```python
from build123d import *

# Parameters (mm, degrees)
SKETCH_1_R          = 3.2
SKETCH_1_R_2        = 1.8
SKETCH_1_R_3        = 5.7
SKETCH_1_R_4        = 1.7
EXTRUDE_1_DEPTH     = 3
SKETCH_2_R          = 10.5
EXTRUDE_2_DEPTH     = 7
SKETCH_4_R          = 1.7
CUT_EXTRUDE_1_DEPTH = 7
CUT_EXTRUDE_2_DEPTH = 3.5
SKETCH_6_R          = 5.7
CUT_EXTRUDE_3_DEPTH = 20
SKETCH_7_R          = 5
SKETCH_7_R_2        = 3.2
EXTRUDE_3_DEPTH     = 15
SKETCH_8_W          = 10
SKETCH_8_H          = 4
SKETCH_8_W_2        = 4
SKETCH_8_H_2        = 6
EXTRUDE_4_DEPTH     = 15
CUT_EXTRUDE_4_DEPTH = 15
CUT_EXTRUDE_5_DEPTH = 15
CUT_EXTRUDE_6_DEPTH = 15
SKETCH_12_W         = 25.575378798
SKETCH_12_H         = 2.842045507
EXTRUDE_5_DEPTH     = 7


with BuildPart() as part:
    # 草图1 → 凸台-拉伸1 (new body)
    with BuildSketch(Plane(origin=(0, 0, 0), x_dir=(1, 0, 0), z_dir=(0, 1, 0))):
        with BuildLine():
            Line((-35.081832586, -10), (-40, -10))
            Line((-40, -10), (-40, 10))
            Line((-40, 10), (-11.180339887, 10))
            ThreePointArc((-11.180339887, 10), (0, 15), (11.180339887, 10))
            Line((11.180339887, 10), (40, 10))
            Line((40, 10), (40, -10))
            Line((40, -10), (20, -10))
            Line((20, -10), (43.844622395, -33.844622395))
            Line((43.844622395, -33.844622395), (33.844622395, -43.844622395))
            Line((33.844622395, -43.844622395), (10, -20))
            Line((10, -20), (-10, -20))
            Line((-10, -20), (-33.713203436, -43.713203436))
            Line((-33.713203436, -43.713203436), (-43.713203436, -33.713203436))
            Line((-43.713203436, -33.713203436), (-20, -10))
            Line((-20, -10), (-35.081832586, -10))
        make_face()
        with Locations((35, 0)):
            Circle(SKETCH_1_R, mode=Mode.SUBTRACT)
        with Locations((-15.5, -15.5)):
            Circle(SKETCH_1_R_2, mode=Mode.SUBTRACT)
        with Locations((15.5, -15.5)):
            Circle(SKETCH_1_R_2, mode=Mode.SUBTRACT)
        with Locations((-35, 0)):
            Circle(SKETCH_1_R, mode=Mode.SUBTRACT)
        Circle(SKETCH_1_R_3, mode=Mode.SUBTRACT)
        with Locations((-8, 0)):
            Circle(SKETCH_1_R_4, mode=Mode.SUBTRACT)
        with Locations((0, 8)):
            Circle(SKETCH_1_R_4, mode=Mode.SUBTRACT)
        with Locations((8, 0)):
            Circle(SKETCH_1_R_4, mode=Mode.SUBTRACT)
        with Locations((0, -8)):
            Circle(SKETCH_1_R_4, mode=Mode.SUBTRACT)
        with BuildLine():
            Line((-18.818376618, -21.081118318), (-35.081832586, -37.344574285))
            ThreePointArc((-35.081832586, -37.344574285), (-37.344574285, -37.344574285), (-37.344574285, -35.081832586))
            Line((-37.344574285, -35.081832586), (-21.081118318, -18.818376618))
            ThreePointArc((-21.081118318, -18.818376618), (-18.818376618, -18.818376618), (-18.818376618, -21.081118318))
        make_face(mode=Mode.SUBTRACT)
        with BuildLine():
            Line((21.081118316, -18.818376616), (37.344574284, -35.081832584))
            ThreePointArc((37.344574284, -35.081832584), (37.344574284, -37.344574284), (35.081832584, -37.344574284))
            Line((35.081832584, -37.344574284), (18.818376616, -21.081118316))
            ThreePointArc((18.818376616, -21.081118316), (18.818376616, -18.818376616), (21.081118316, -18.818376616))
        make_face(mode=Mode.SUBTRACT)
    extrude(amount=EXTRUDE_1_DEPTH)

    # 草图2 → 凸台-拉伸2 (add)
    with BuildSketch(Plane(origin=(0, 3, 0), x_dir=(1, 0, 0), z_dir=(0, 1, 0))):
        Circle(SKETCH_2_R)
    extrude(amount=EXTRUDE_2_DEPTH)

    # 草图4 → 切除-拉伸1 (cut)
    with BuildSketch(Plane.XZ.offset(-3)):
        with Locations((0, -8)):
            Circle(SKETCH_4_R)
        with Locations((-8, 0)):
            Circle(SKETCH_4_R)
        with Locations((8, 0)):
            Circle(SKETCH_4_R)
        with Locations((0, 8)):
            Circle(SKETCH_4_R)
    extrude(amount=-CUT_EXTRUDE_1_DEPTH, mode=Mode.SUBTRACT)

    # 草图5 → 切除-拉伸2 (cut)
    with BuildSketch(Plane(origin=(0, 3, 0), x_dir=(1, 0, 0), z_dir=(0, 1, 0))):
        Polygon((-4.766838493, 0), (-6.383419246, 2.8), (-11.233161507, 2.8), (-11.233161507, -2.8), (-6.383419246, -2.8), align=None)
        Polygon((4.766838493, 0), (6.383419246, -2.8), (11.233161507, -2.8), (11.233161507, 2.8), (6.383419246, 2.8), align=None)
        Polygon((-2.8, 11.233161507), (-2.8, 6.383419246), (0, 4.766838493), (2.8, 6.383419246), (2.8, 11.233161507), align=None)
        Polygon((0, -4.766838493), (-2.8, -6.383419246), (-2.8, -11.233161507), (2.8, -11.233161507), (2.8, -6.383419246), align=None)
    extrude(amount=CUT_EXTRUDE_2_DEPTH, mode=Mode.SUBTRACT)

    # 草图6 → 切除-拉伸3 (cut)
    with BuildSketch(Plane.XZ.offset(-3)):
        Circle(SKETCH_6_R)
    extrude(amount=-CUT_EXTRUDE_3_DEPTH, mode=Mode.SUBTRACT)

    # 草图7 → 凸台-拉伸3 (add)
    with BuildSketch(Plane(origin=(0, 3, 0), x_dir=(1, 0, 0), z_dir=(0, 1, 0))):
        with Locations((-35, 0)):
            Circle(SKETCH_7_R)
        with Locations((-35, 0)):
            Circle(SKETCH_7_R_2, mode=Mode.SUBTRACT)
        with Locations((35, 0)):
            Circle(SKETCH_7_R)
        with Locations((35, 0)):
            Circle(SKETCH_7_R_2, mode=Mode.SUBTRACT)
    extrude(amount=EXTRUDE_3_DEPTH)

    # 草图8 → 凸台-拉伸4 (add)
    with BuildSketch(Plane(origin=(0, 3, 0), x_dir=(1, 0, 0), z_dir=(0, 1, 0))):
        with Locations((-26, 0)):
            Rectangle(SKETCH_8_W, SKETCH_8_H)
        with Locations((-35, 7)):
            Rectangle(SKETCH_8_W_2, SKETCH_8_H_2)
        with Locations((-35, -7)):
            Rectangle(SKETCH_8_W_2, SKETCH_8_H_2)
        with Locations((26, 0)):
            Rectangle(SKETCH_8_W, SKETCH_8_H)
        with Locations((35, 7)):
            Rectangle(SKETCH_8_W_2, SKETCH_8_H_2)
        with Locations((35, -7)):
            Rectangle(SKETCH_8_W_2, SKETCH_8_H_2)
    extrude(amount=EXTRUDE_4_DEPTH)

    # 草图9 → 切除-拉伸4 (cut)
    with BuildSketch(Plane.XY.offset(2)):
        Polygon((-30.417424305, 18), (-21, 3), (-21, 18), align=None)
        Polygon((21, 3), (30.417424305, 18), (21, 18), align=None)
    extrude(amount=-CUT_EXTRUDE_4_DEPTH, mode=Mode.SUBTRACT)

    # 草图10 → 切除-拉伸5 (cut)
    with BuildSketch(Plane.ZY.offset(-33)):
        Polygon((-4.582575695, 18), (-10, 3), (-10, 18), align=None)
        Polygon((4.582575695, 18), (10, 18), (10, 3), align=None)
    extrude(amount=-CUT_EXTRUDE_5_DEPTH, mode=Mode.SUBTRACT)

    # 草图11 → 切除-拉伸6 (cut)
    with BuildSketch(Plane(origin=(-33, 0, 0), x_dir=(0, 0, -1), z_dir=(1, 0, 0))):
        Polygon((-4.582575695, 18), (-10, 3), (-10, 18), align=None)
        Polygon((4.582575695, 18), (10, 3), (10, 18), align=None)
    extrude(amount=-CUT_EXTRUDE_6_DEPTH, mode=Mode.SUBTRACT)

    # 草图12 → 凸台-拉伸5 (add)
    with BuildSketch(Plane(origin=(0, 3, 0), x_dir=(1, 0, 0), z_dir=(0, 1, 0))):
        with Locations((-20.212310601, -6.003598449)):
            Rectangle(SKETCH_12_W, SKETCH_12_H)
        with Locations((-20.212310601, 6.003598449)):
            Rectangle(SKETCH_12_W, SKETCH_12_H)
        with Locations((20.212310601, 6.003598449)):
            Rectangle(SKETCH_12_W, SKETCH_12_H)
        with Locations((20.212310601, -6.003598449)):
            Rectangle(SKETCH_12_W, SKETCH_12_H)
    extrude(amount=EXTRUDE_5_DEPTH)


solid = part.part
```
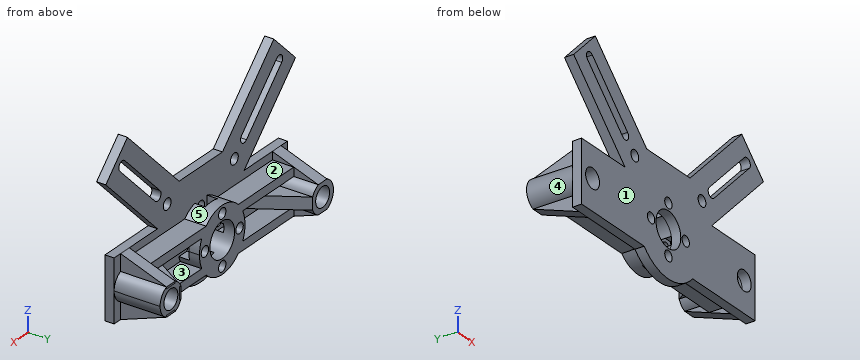
CAD build for the part. Positions are in the model's coordinates, mm. Face numbers are marked on the shaded views. A direction names the side the tool comes from. Round coordinates to 2 decimals unless told otherwise and drop trailing zeros. Write each loop counter-clockwise with the first axis right and the second up, starting at its lowest first coordinate (ties: lowest second). Pieces come first, ordered by that corner, then holes. Notation, with made-up numbers: (26, 1) -> (40, 1) arc R17 ccw to (40, 12) -> close; hole circle Ø9 at (44, 36.5). An arc over 180 degrees is marked (long way). Answer in a Markdown table with one row per item. Add a question column.
Item 1: Saw through at B-B, the plane y = 15. Write the cut outline in (x, z).
Item 2: Mould opens along Z. For the marked faces 3, 4 and 5 say: pulls with the +Z half, pulls with the -Z half, needs draft (parallel to the pull), parting line crosses it, or undercut.
Item 3: Saw through at D-D, the plane x = 27.5. Write the cut outline in (y, z).
Item 4: Saw through at A-A, the plane x = -15.5. Write the cut outline in (y, z).
Item 5: Drop flat-ended pins along their axis: pin 1 Ø8 at (x, y) = (33.5, 2.5) entering from -Z; pin 2 Ø10 at (x, z) = (-27, 17) entering from +Y; pin 3 Ø4 at (x, z) = (0, 8) entering from -Y; pin 4 Ø4.5 at (y, z) = (7, -7) entering from +X. Give the stop position or say it passes through.
Item 6: Saw through at C-C, the plane z = 29.5. Write the cut outline in (x, y).
Item 7: Drill centre lines: line 1 (Z direction, x = 29, y = 3.25); line 2 (X direction, y = 2.35, z = 0); line 3 (Y direction, x = 9, z = 2). Where is each one in solid material? Low to high. Write a range as from..to.
Item 8: Which spindle directions (+Z, -Z, +X, -X, +Y, -Y) get a long thin tool onto all of the face, cutting with end or side? Do the marked faces 1 and 2. Say none if no direction does.
Findings below:
| question | item | result |
|---|---|---|
| 1 | outline | (-37, -5.67) -> (-33, -5.67) -> (-33, -4.58) arc R5 ccw to (-30.42, -2) -> (-28.53, -2) -> (-28.53, 2) -> (-30.42, 2) arc R5 ccw to (-33, 4.58) -> (-33, 5.67) -> (-37, 5.67) -> (-37, 4.58) arc R5 ccw to (-37, -4.58) -> close; (28.53, -2) -> (30.42, -2) arc R5 ccw to (33, -4.58) -> (33, -5.67) -> (37, -5.67) -> (37, -4.58) arc R5 ccw to (37, 4.58) -> (37, 5.67) -> (33, 5.67) -> (33, 4.58) arc R5 ccw to (30.42, 2) -> (28.53, 2) -> close; hole circle Ø6.4 at (-35, 0); hole circle Ø6.4 at (35, 0) |
| 2 | face 3 | undercut |
| 2 | face 4 | parting line crosses it |
| 2 | face 5 | pulls with the +Z half |
| 3 | outline | (0, -10) -> (3, -10) -> (3, -7.42) -> (10, -7.42) -> (10, -4.58) -> (3, -4.58) -> (3, -2) -> (13.35, -2) -> (13.35, 2) -> (3, 2) -> (3, 4.58) -> (10, 4.58) -> (10, 7.42) -> (3, 7.42) -> (3, 10) -> (0, 10) -> close; (0, 17.5) -> (3, 17.5) -> (3, 25.24) -> (0, 25.24) -> close; (0, 29.76) -> (3, 29.76) -> (3, 37.5) -> (0, 37.5) -> close |
| 4 | outline | (0, -10) -> (3, -10) -> (3, -7.42) -> (10, -7.42) -> (10, -4.58) -> (3, -4.58) -> (3, 4.58) -> (10, 4.58) -> (10, 7.42) -> (3, 7.42) -> (3, 13.7) -> (0, 13.7) -> close; (0, 17.3) -> (3, 17.3) -> (3, 25.5) -> (0, 25.5) -> close |
| 5 | pin 1 | stops at z = -10 |
| 5 | pin 2 | stops at y = 3 |
| 5 | pin 3 | stops at y = 0 |
| 5 | pin 4 | stops at x = 37 |
| 6 | outline | (-39.5, 0) -> (-31.76, 0) -> (-31.76, 3) -> (-39.5, 3) -> close; (-27.24, 0) -> (-19.5, 0) -> (-19.5, 3) -> (-27.24, 3) -> close; (19.5, 0) -> (27.24, 0) -> (27.24, 3) -> (19.5, 3) -> close; (31.76, 0) -> (39.5, 0) -> (39.5, 3) -> (31.76, 3) -> close |
| 7 | line 1 | z = -7.42..-4.58, -2..2, 4.58..7.42 |
| 7 | line 2 | x = -40..-38.2, -31.8..-9.7, -6.3..-5.7, 5.7..6.3, 9.7..31.8, 38.2..40 |
| 7 | line 3 | y = 0..3, 6.5..10 |
| 8 | face 1 | +Z, -Z, +X, -X, -Y |
| 8 | face 2 | +Z, +Y |
